from build123d import *

# Parameters (mm, degrees)
SKETCH_1_W           = 15
SKETCH_1_H           = 15
EXTRUDE_1_DEPTH      = 2
SKETCH_2_R           = 3
EXTRUDE_2_DEPTH      = 1
SKETCH_3_R           = 2
EXTRUDE_3_DEPTH      = 10
SKETCH_5_W           = 1
SKETCH_5_H           = 6
CUT_EXTRUDE_1_DEPTH  = 6
EXTRUDE_4_DEPTH      = 7.5
EXTRUDE_4_DEPTH_BACK = 7.5
FILLET_1_R           = 0.2
FILLET_2_R           = 0.1


with BuildPart() as part:
    # Sketch 1 → Extrude 1 (new body)
    with BuildSketch(Plane(origin=(0, 0, 0), x_dir=(1, 0, 0), z_dir=(0, 1, 0))):
        Rectangle(SKETCH_1_W, SKETCH_1_H)
    extrude(amount=EXTRUDE_1_DEPTH)

    # Sketch 2 → Extrude 2 (add)
    with BuildSketch(Plane(origin=(0, 2, 0), x_dir=(1, 0, 0), z_dir=(0, 1, 0))):
        with Locations(Location((0, 0, 0), (0, 0, 90))):
            Circle(SKETCH_2_R)
    extrude(amount=EXTRUDE_2_DEPTH)

    # Sketch 3 → Extrude 3 (add)
    with BuildSketch(Plane(origin=(0, 3, 0), x_dir=(1, 0, 0), z_dir=(0, 1, 0))):
        with Locations(Location((0, 0, 0), (0, 0, 270))):
            Circle(SKETCH_3_R)
    extrude(amount=EXTRUDE_3_DEPTH)

    # Sketch 4 → Revolve 1 (revolve)
    with BuildSketch(Plane.XY, mode=Mode.PRIVATE) as revolve_1_sk:
        Polygon((0, 13), (-2, 13), (-2.1, 12), (0, 12), align=None)
    revolve(revolve_1_sk.sketch.rotate(Axis((0, 12, 0), (0, 1, 0)), 90), axis=Axis((0, 12, 0), (0, 1, 0)))

    # Sketch 5 → Cut-Extrude 1 (cut)
    with BuildSketch(Plane(origin=(0, 13, 0), x_dir=(1, 0, 0), z_dir=(0, 1, 0))):
        Rectangle(SKETCH_5_W, SKETCH_5_H)
    extrude(amount=-CUT_EXTRUDE_1_DEPTH, mode=Mode.SUBTRACT)

    # Sketch 6 → Extrude 4 (add, two sides: drawn at the far end of the back side and taken through both)
    with BuildSketch(Plane.XY.offset(-EXTRUDE_4_DEPTH_BACK)):
        with BuildLine():
            Line((-0.5, 0), (-1.5, 0))
            Line((-1.5, 0), (-1.5, -0.677124344))
            ThreePointArc((-1.5, -0.677124344), (-1.780042303, -1.088161527), (-1.95, -1.555590279))
            Line((-1.95, -1.555590279), (-1.95, -2.5))
            Line((-1.95, -2.5), (-1.165769145, -2.5))
            Line((-1.165769145, -2.5), (-0.5, -1.07225346))
            Line((-0.5, -1.07225346), (-0.5, 0))
        make_face()
        with BuildLine():
            Line((0.5, 0), (0.5, -1.07225346))
            Line((0.5, -1.07225346), (1.165769145, -2.5))
            Line((1.165769145, -2.5), (1.95, -2.5))
            Line((1.95, -2.5), (1.95, -1.555590279))
            ThreePointArc((1.95, -1.555590279), (1.780042303, -1.088161527), (1.5, -0.677124344))
            Line((1.5, -0.677124344), (1.5, 0))
            Line((1.5, 0), (0.5, 0))
        make_face()
    extrude(amount=EXTRUDE_4_DEPTH + EXTRUDE_4_DEPTH_BACK)

    # Fillet 1
    fillet_1_edges = [part.edges().sort_by_distance(p)[0] for p in [
        (-7.5, 1, -7.5),
        (7.5, 1, -7.5),
        (7.5, 1, 7.5),
        (-7.5, 1, 7.5),
        (7.5, 2, 0),
        (0, 2, -7.5),
        (-7.5, 2, 0),
        (0, 2, 7.5),
        (0, 3, 3),
    ]]
    fillet(fillet_1_edges, radius=FILLET_1_R)

    # Fillet 2
    fillet_2_edges = [part.edges().sort_by_distance(p)[0] for p in [
        (-1.165769145, -2.5, 0),
        (-1.95, -2.5, 0),
        (1.95, -2.5, 0),
        (1.165769145, -2.5, 0),
    ]]
    fillet(fillet_2_edges, radius=FILLET_2_R)


solid = part.part
Verification items for the finished model (mm, model axes). A direction names the side the tool comes from. Round coordinates to 2 decimals unless told otherwise and drop trailing zeros. Loops run counter-clockwise (first coordinate to the right, second up) from the corner with the lowest first, then second, coordinate; pieces in that order, holes last. Notation, with made-up numbers: (-40, -11) - (-11, -11) arc R29 ccw to (-11, 22) - close; hole circle Ø3 at (83, 61). An arc over 180 degrees is marked (long way). Use one line per item in the form item = value.
1. Access from +Z, -Z, +X, -X, +Y, -Y to the whole of each face (thin tool, end or side, straight path). Record for faces 5 (the flat face through (1.95, -2, 0)), 6 (the flat face through (0.5, 10, 0)), 7 (the cylindrical face through (-1.777, -1.082, -0.105)), 8 (the flat face through (0.5, -0.5, -0.1)), 9 (the cylindrical face through (-0.766, 7.437, 1.847)).
A:
face_5 = +Z, -Z, +X, -Y
face_6 = +Z, -Z, +Y
face_7 = +Z, -Z, -X
face_8 = +Z, -Z, -Y
face_9 = none
2. Section check C-C on z = 6.75. Record the cut outline in (x, y).
A:
outline = (-7.5, 0) - (-1.5, 0) - (-1.5, -0.68) arc R2 ccw to (-1.95, -1.56) - (-1.95, -2.4) arc R0.1 ccw to (-1.85, -2.5) - (-1.23, -2.5) arc R0.1 ccw to (-1.14, -2.44) - (-0.5, -1.07) - (-0.5, 0) - (0.5, 0) - (0.5, -1.07) - (1.14, -2.44) arc R0.1 ccw to (1.23, -2.5) - (1.85, -2.5) arc R0.1 ccw to (1.95, -2.4) - (1.95, -1.56) arc R2 ccw to (1.5, -0.68) - (1.5, 0) - (7.5, 0) - (7.5, 1.8) arc R0.2 ccw to (7.3, 2) - (-7.3, 2) arc R0.2 ccw to (-7.5, 1.8) - close
3. Scan lines: probe 1 along X at (y, z) = (9.5, 0.75); probe 2 along Y at (x, z) = (-5, -6.75); probe 3 along X at (y, z) = (-1.5, 5.75). Record each from-to range of solid material in increasing order.
A:
probe_1 = -1.85 to -0.5, 0.5 to 1.85
probe_2 = 0 to 2
probe_3 = -1.94 to -0.7, 0.7 to 1.94
4. Gauge pin test, flat ends, axial feed: pin 1 Ø1 at (x, z) = (4, 0) entering from -Y; pin 2 Ø4 at (y, z) = (5, 5.5) entering from -X; pin 3 Ø8 at (y, z) = (9, 4.5) entering from +X; pin 4 Ø3.5 at (y, z) = (9, 0) entering from +X. Record the tip position at first contact, or that the pin passes through.
A:
pin_1 = 0
pin_2 = through
pin_3 = 1.94
pin_4 = 2
5. Section check A-A on y = -0.25. Record the cut outline in (x, z).
A:
outline = (-1.5, -7.5) - (-0.5, -7.5) - (-0.5, 7.5) - (-1.5, 7.5) - close; (0.5, -7.5) - (1.5, -7.5) - (1.5, 7.5) - (0.5, 7.5) - close
6. Section check B-B on x = 0. Record the cut outline in (y, z).
A:
outline = (0, -7.5) - (1.8, -7.5) arc R0.2 ccw to (2, -7.3) - (2, -3) - (2.8, -3) arc R0.2 ccw to (3, -2.8) - (3, -2) - (7, -2) - (7, 2) - (3, 2) - (3, 2.8) arc R0.2 ccw to (2.8, 3) - (2, 3) - (2, 7.3) arc R0.2 ccw to (1.8, 7.5) - (0, 7.5) - close
7. Draft check along X on faces 1 (the flat face through (0, 0, 0)), 2 (the flat face through (-7.5, 1, 0)), 3 (the cylindrical face through (1.78, -1.09, -0.11)), 4 (the flat face through (-0.5, -0.5, -0.1)). Enter one of: pulls with the +X half, pulls with the -X half, needs draft (parallel to the pull), parting line crosses it, or undercut.
A:
face_1 = undercut
face_2 = pulls with the -X half
face_3 = pulls with the +X half
face_4 = undercut
8. Section check D-D on y = 4.25. Record the cut outline in (x, z).
A:
outline = circle Ø4 at (0, 0)
